The drawing under review shows one solid part. Ordinate dimensions are in mm from its lowest x, y, z. A direction names the side the tool comes from. Give positions to 0.01 mm unless a question says otherwise; leave off trailing zeros. Loops run counter-clockwise (first coordinate to the right, second up) from the corner with the lowest first, then second, coordinate; pieces in that order, holes last. Notation, with made-up numbers: M 36.25,32 L 77.25,32 A7 ccw 77.25,38 Z; hole C 20.5,68 d2. An arc over 180 degrees is marked long. Write item = value, one per line. Start each with the question number.
1. For the marked faces 1, 2 and 3, list the 3-axis set-ups (+Z, -Z, +X, -X, +Y, -Y) from which the entire face can be reached by the end or side of a thin tool; tool diameter is ignored.
2. We need section B-B on y = 12. Give the boundary of the cut face in (x, z), then the cut area to 3 significant figures.
3. Draft analysis for pull direction Z (two halves, no side actions). For the marked faces 4, 5 and 6, state which applies: pulls with the +Z half, pulls with the -Z half, needs draft (parallel to the pull), parting line crosses it, or undercut.
4. Wall thickness on line 1 along X through (y, z) = (8.75, 3); line 2 along X through (y, z) = (12.5, 27.5); line 3 along Z through (x, y) = (16.5, 18.5): over which ranges is each line inside the solid? List them lowest first. Write a range as from..to.
5. We need section A-A on z = 10.75. Give the boundary of the cut face in (x, y), then the cut area to 3 significant figures.
6. We need section C-C on y = 23. Give the boundary of the cut face in (x, z).
7. We need section D-D on x = 4. Give the boundary of the cut face in (y, z) (3 decimals), then the cut area to 3 significant figures.
8. For pin 1 (1.5 mm diameter, centred on x = 6, y = 17.5, fed in from -Z); pin 2 (4 mm diameter, centred on x = 20, y = 26.5, fed in from +Z); pin 3 (9 mm diameter, centred on y = 14.935, z = 14.935, fed in from -X); pin 4 (2 mm diameter, centred on x = 11.5, y = 15, fed in from +Z), all flat-tipped, find the tip position at first contact; note any pin that passes through.
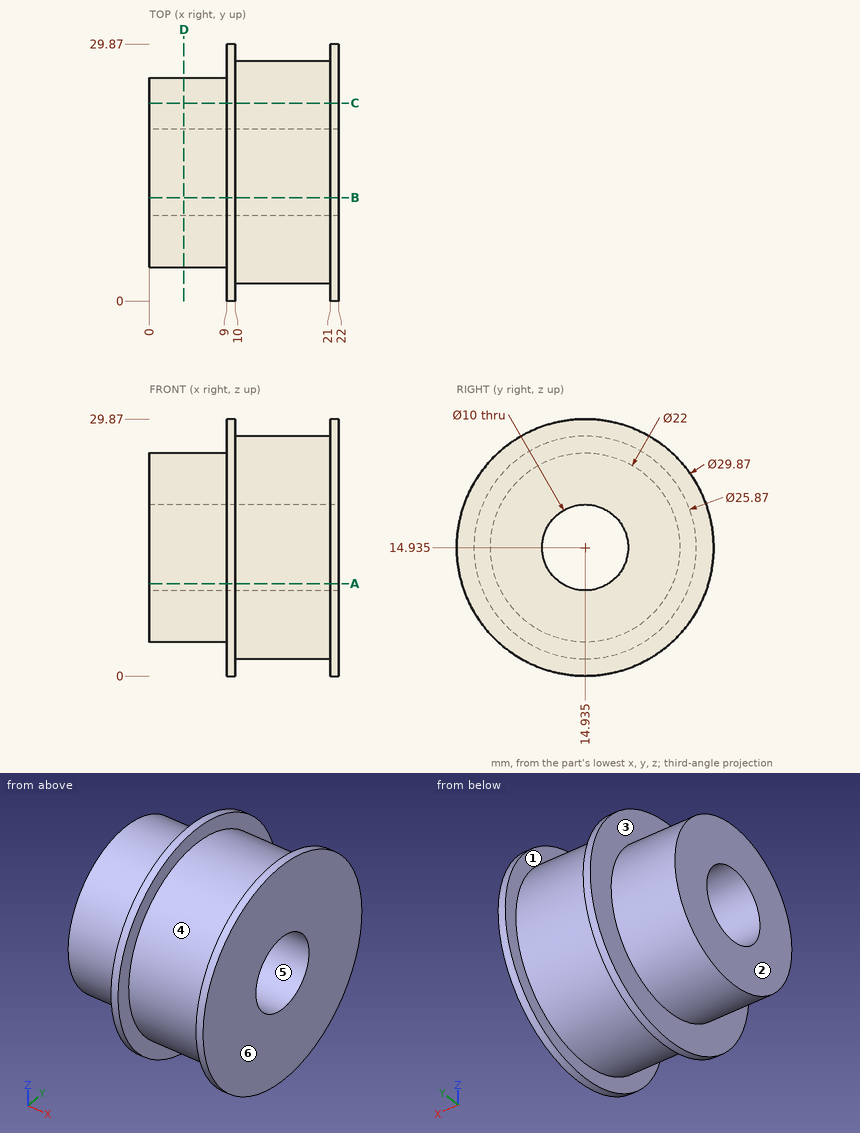
Final values:
q1.face_1 = none
q1.face_2 = +Z, -Z, -X, +Y, -Y
q1.face_3 = -X
q2.outline = M 0,4.33 L 9,4.33 L 9,0.29 L 10,0.29 L 10,2.34 L 21,2.34 L 21,0.29 L 22,0.29 L 22,10.89 L 0,10.89 Z; M 0,18.98 L 22,18.98 L 22,29.58 L 21,29.58 L 21,27.53 L 10,27.53 L 10,29.58 L 9,29.58 L 9,25.54 L 0,25.54 Z
q2.area = 348 mm²
q3.face_4 = parting line crosses it
q3.face_5 = undercut
q3.face_6 = needs draft
q4.line_1 = 9..10, 21..22
q4.line_2 = 9..22
q4.line_3 = 2.5..11.43, 18.44..27.37
q5.outline = M 0,4.76 L 9,4.76 L 9,0.6 L 10,0.6 L 10,2.7 L 21,2.7 L 21,0.6 L 22,0.6 L 22,12.2 L 0,12.2 Z; M 0,17.67 L 22,17.67 L 22,29.27 L 21,29.27 L 21,27.17 L 10,27.17 L 10,29.27 L 9,29.27 L 9,25.11 L 0,25.11 Z
q5.area = 389 mm²
q6.outline = M 0,7.45 L 9,7.45 L 9,2.36 L 10,2.36 L 10,4.82 L 21,4.82 L 21,2.36 L 22,2.36 L 22,27.51 L 21,27.51 L 21,25.05 L 10,25.05 L 10,27.51 L 9,27.51 L 9,22.42 L 0,22.42 Z
q7.outline = C 14.935,14.935 d22; hole C 14.935,14.935 d10
q7.area = 302 mm²
q8.pin_1 = 4.09
q8.pin_2 = 26.18
q8.pin_3 = through
q8.pin_4 = 27.87
